The model under review builds one solid part; all positions refer to its coordinate system, in mm. A direction names the side the tool comes from. Round coordinates to 2 decimals unless told otherwise and drop trailing zeros. Order: outer loops, then holes, each group sorted by start corner. A loop starts at its lowest first (then second) coordinate and runs counter-clockwise, first axis right, second up. Notation, with made-up numbers: (51, 17) -> (110, 17) arc R19 cw to (110, 39) -> close; hole circle Ø3 at (5, 51). An arc over 180 degrees is marked (long way). Put each result on its own line as item: value. Start each with the question number.
Autodesk Inventor part; units mm, degrees
ref_plane "YZ Plane" through (0, 0, 0) normal (1, 0, 0) x (0, 1, 0)
ref_plane "XZ Plane" through (0, 0, 0) normal (0, 1, 0) x (-1, 0, 0)
ref_plane "XY Plane" through (0, 0, 0) normal (0, 0, 1) x (1, 0, 0)
sketch "Sketch1" plane through (0, 0, 0) normal (0, 1, 0) x (-1, 0, 0)
  line L0 (-6.6675, 1.5875) -> (6.6675, 1.5875)
  line L1 (6.6675, 1.5875) -> (6.6675, -1.5875)
  line L2 (6.6675, -1.5875) -> (-6.6675, -1.5875)
  line L3 (-6.6675, -1.5875) -> (-6.6675, 1.5875)
  point P0 (0, 0)
  dimension "d0" = 13.335
  dimension "d1" = 3.175
  dimension "d2" = 1.5875
  dimension "d3" = 6.6675
extrude "Extrusion1" add sketch "Sketch1" along normal blind 12.7
sketch "Sketch2" plane through (0, 12.7, 0) normal (0, 1, 0) x (1, 0, 0)
  line L0 (6.6675, -1.5875) -> (6.6675, 1.5875)
  line L1 (6.6675, 1.5875) -> (-6.6675, 1.5875)
  line L2 (-6.6675, 1.5875) -> (-6.6675, -1.5875)
  line L3 (-6.6675, -1.5875) -> (-0.9525, -1.5875)
  line L4 (-0.9525, -1.5875) -> (-0.9525, 1.5875)
  line L5 (-0.9525, 1.5875) -> (-6.6675, 1.5875)
  line L6 (-6.6675, 1.5875) -> (-6.6675, -1.5875)
  line L7 (6.6675, -1.5875) -> (0.9525, -1.5875)
  line L8 (0.9525, -1.5875) -> (0.9525, 1.5875)
  line L9 (0.9525, 1.5875) -> (6.6675, 1.5875)
  line L10 (6.6675, 1.5875) -> (6.6675, -1.5875)
  point P0 (0, 0)
  dimension "d6" = 5.715
  dimension "d7" = 5.715
extrude "Extrusion2" add sketch "Sketch2" along normal blind 7.62
sketch "Sketch3" plane through (6.6675, 0, 1.5875) normal (1, 0, 0) x (0, 0, -1)
  line L0 (3.175, 0) -> (0, 0)
  line L1 (3.175, 0) -> (3.175, 20.32)
  line L2 (0, 0) -> (3.175, 0)
  line L3 (3.175, 0) -> (3.175, 12.7)
  line L4 (3.175, 12.7) -> (0, 12.7)
  line L5 (0, 12.7) -> (0, 0)
  point P0 (1.5875, 0)
  dimension "d10" = 0
  dimension "d11" = 12.7
extrude "Extrusion3" add sketch "Sketch3" along normal blind 6.35
sketch "Sketch4" plane through (-6.6675, 0, -1.5875) normal (-1, 0, 0) x (0, 0, 1)
  line L0 (0, 0) -> (3.175, 0)
  line L1 (3.175, 0) -> (3.175, 12.7)
  line L2 (3.175, 12.7) -> (0, 12.7)
  line L3 (0, 12.7) -> (0, 0)
  point P0 (1.5875, 0)
  dimension "d14" = 3.175
  dimension "d15" = 12.7
extrude "Extrusion4" add sketch "Sketch4" along normal blind 6.35
sketch "Sketch5" plane through (0.9525, 20.32, 1.5875) normal (0, 0, 1) x (1, 0, 0)
  line L0 (-13.97, -20.32) -> (12.065, -20.32)
  line L1 (12.065, -20.32) -> (12.065, -17.145)
  line L2 (12.065, -17.145) -> (-13.97, -17.145)
  line L3 (-13.97, -17.145) -> (-13.97, -20.32)
  point P0 (-0.9525, -20.32)
  dimension "d18" = 26.035
  dimension "d19" = 3.175
extrude "Extrusion5" add sketch "Sketch5" along normal blind 3.175
fillet "Fillet1" radius 3.175 3 edges at (0, 3.175, 4.7625) (0, 3.175, 1.5875) (0, 0, 4.7625)
equation "\"d7\" = d6"
properties part number "batteryFalg"
Q1. Take a section at A-A on y = 18.5. Give the boundary of the cut face in (x, z), and give its area (3 significant figures).
Q2. Wall thickness on probe 1 along X at (y, z) = (17.5, -1.3); probe 2 along Z at (x, y) = (3.5, 17); probe 3 along Y at (x, z) = (11, -0.55): over which ranges is each line inside the solid? List them lowest first. Write a range as [from, to].
Q3. Draft analysis for pull direction X (two halves, no side actions). For faces 6 (the face through (-6.668, 16, 0)), 7 (the face through (0, 0, -1)), 8 (the face through (0.952, 16, 0)), state which applies: +X half, -X half, draft (parallel to the pull), parting line (faces both ways), or undercut.
Q4. Take a section at C-C on z = 0.95. Give the boundary of the cut face in (x, y), and give its area (3 significant figures).
Q5. Clearance check with flat-ended pins moving along their axes: pin 1 Ø4 at (x, y) = (4.5, 16) entering from +Z; pin 2 Ø1 at (y, z) = (15, -0.5) entering from +X; pin 3 Ø1.5 at (x, z) = (-9.5, 1) entering from +Y; pin 4 Ø8 at (x, y) = (7.5, 5.5) entering from +Z. State where each tip first meets the part, or that it passes through.
Q6. For faces 1 (the face through (0, 12.7, 0)), 2 (the face through (0, 12, 1.588)), 3 (the face through (6.668, 16, 0)), 4 (the face through (-10, 12.7, 0)), 5 (the face through (-13.018, 6, 0)), list the 3-axis set-ups (+Z, -Z, +X, -X, +Y, -Y) from which the entire face can be reached by the end or side of a thin tool; tool diameter is ignored.
Q7. Take a section at D-D on y = 7.5. Give the boundary of the cut face in (x, z), and give its area (3 significant figures).
Calculated:
1. outline: (-6.67, -1.59) -> (-0.95, -1.59) -> (-0.95, 1.59) -> (-6.67, 1.59) -> close; (0.95, -1.59) -> (6.67, -1.59) -> (6.67, 1.59) -> (0.95, 1.59) -> close
1. area: 36.3 mm²
2. probe 1: x = [-6.67, -0.95], [0.95, 6.67]
2. probe 2: z = [-1.59, 1.59]
2. probe 3: y = [0.01, 12.7]
3. face 6: -X half
3. face 7: draft
3. face 8: undercut
4. outline: (-13.02, 0.49) -> (13.02, 0.49) -> (13.02, 12.7) -> (6.67, 12.7) -> (6.67, 20.32) -> (0.95, 20.32) -> (0.95, 12.7) -> (-0.95, 12.7) -> (-0.95, 20.32) -> (-6.67, 20.32) -> (-6.67, 12.7) -> (-13.02, 12.7) -> close
4. area: 405 mm²
5. pin 1: stops at z = 1.59
5. pin 2: stops at x = 6.67
5. pin 3: stops at y = 12.7
5. pin 4: stops at z = 2.44
6. face 1: +Z, -Z, +Y
6. face 2: +Z, +X, -X, +Y
6. face 3: +Z, -Z, +X, +Y
6. face 4: +Z, -Z, -X, +Y
6. face 5: +Z, -Z, -X, +Y, -Y
7. outline: (-13.02, -1.59) -> (13.02, -1.59) -> (13.02, 1.59) -> (-13.02, 1.59) -> close
7. area: 82.7 mm²
